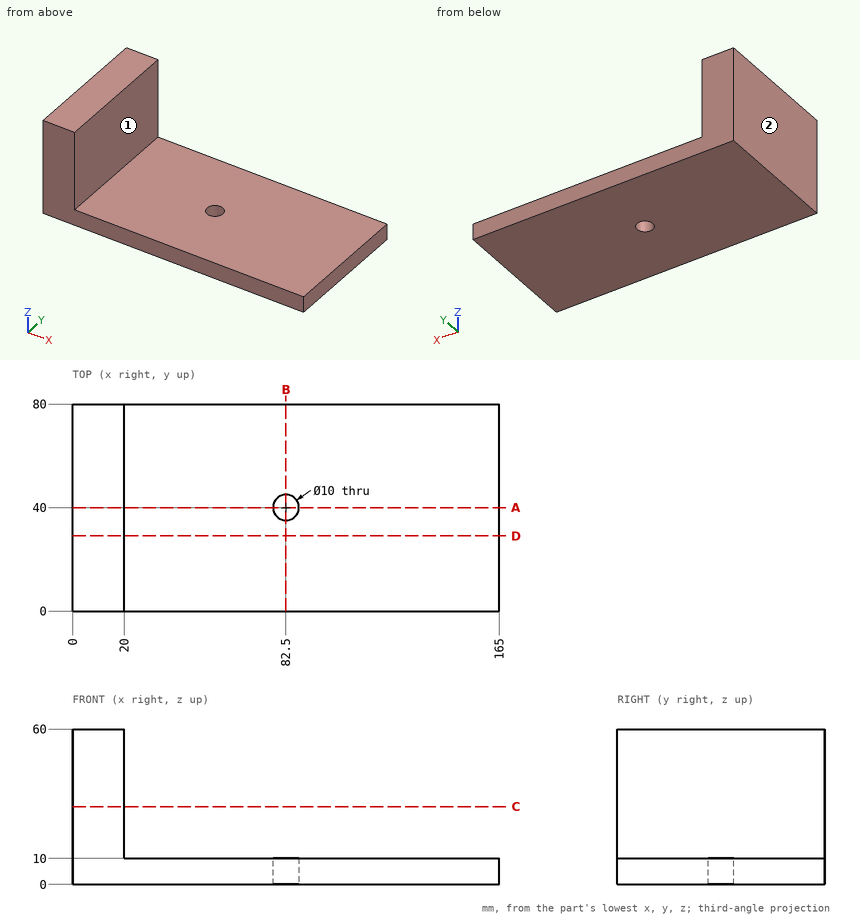
Part print with two shaded views. Sizes in mm from the minimum x, y, z corner. A direction names the side the tool comes from. Give positions to 0.01 mm unless a question says otherwise; leave off trailing zeros. Order: outer loops, then holes, each group sorted by start corner. A loop starts at its lowest first (then second) coordinate and runs counter-clockwise, first axis right, second up.
1) Pin check, flat tips, straight feed: pin 1 (4 mm diameter, centred on y = 69.5, z = 43, fed in from -X); pin 2 (12 mm diameter, centred on x = 110.5, z = 18, fed in from -Y); pin 3 (12 mm diameter, centred on x = 81, y = 31.5, fed in from +Z); pin 4 (3 mm diameter, centred on y = 57.5, z = 21.5, fed in from +X). Stop position of each tip, or through.
2) 3-axis set-ups, long thin cutter, end or side, ignore diameter. For the marked faces 1 and 2: which of +Z, -Z, +X, -X, +Y, -Y reach the whole face in a straight line?
3) Wall check: probe 1 along Y at (x, z) = (82.5, 6); probe 2 along X at (y, z) = (52, 23); probe 3 along Z at (x, y) = (121, 37). Give the ranges that are in metal, low to high.
4) Saw through at D-D, the plane y = 29. Write the cut outline in (x, z), then the cut area to 3 significant figures.
5) Saw through at C-C, the plane z = 30. Write the cut outline in (x, y).
6) Saw through at B-B, the plane x = 82.5. Write the cut outline in (y, z).
7) Saw through at A-A, the plane y = 40. Write the cut outline in (x, z).
Computed:
1. pin 1: stops at x = 0
1. pin 2: passes through
1. pin 3: stops at z = 10
1. pin 4: stops at x = 20
2. face 1: +Z, +X, +Y, -Y
2. face 2: +Z, -Z, -X, +Y, -Y
3. probe 1: y = 0 to 35, 45 to 80
3. probe 2: x = 0 to 20
3. probe 3: z = 0 to 10
4. outline: (0, 0) - (165, 0) - (165, 10) - (20, 10) - (20, 60) - (0, 60) - close
4. area: 2,650 mm2
5. outline: (0, 0) - (20, 0) - (20, 80) - (0, 80) - close
6. outline: (0, 0) - (35, 0) - (35, 10) - (0, 10) - close; (45, 0) - (80, 0) - (80, 10) - (45, 10) - close
7. outline: (0, 0) - (77.5, 0) - (77.5, 10) - (20, 10) - (20, 60) - (0, 60) - close; (87.5, 0) - (165, 0) - (165, 10) - (87.5, 10) - close
